Autodesk Inventor part; units mm, degrees
ref_plane "Work Plane1" through (-7, 16.75, 0) normal (0, 1, 0) x (1, 0, 0)
ref_plane "Work Plane2" through (-7, 15.75, 2) normal (0, 1, 0) x (1, 0, 0)
ref_plane "YZ Plane" through (0, 0, 0) normal (1, 0, 0) x (0, 1, 0)
sketch "Sketch1" plane through (0, 0, 0) normal (0, 0, 1) x (1, 0, 0)
  line L0 (-9.8, 0) -> (9.8, 0) construction
  line L1 (0, -20.65) -> (0, 20.65) construction
  line L2 (7, -14.75) -> (-7, -14.75)
  line L3 (-7, -14.75) -> (-7, 14.75)
  line L4 (-7, 14.75) -> (7, 14.75)
  line L5 (7, 14.75) -> (7, -14.75)
  line L6 (7, -14.75) -> (-7, 14.75) construction
  line L7 (-7, -14.75) -> (7, 14.75) construction
  point P0 (0, 0)
  dimension "d0" = 14
  dimension "d1" = 29.5
extrude "Extrusion1" add sketch "Sketch1" along normal blind 2
ref_plane "Work Plane1" through (-7, 16.75, 0) normal (0, 1, 0) x (1, 0, 0)
sketch "Sketch2" plane through (-7, 16.75, 0) normal (0, 1, 0) x (1, 0, 0)
  line L0 (0, 0) -> (14, 0) construction
  line L1 (0, 0) -> (0, -2) construction
  line L2 (14, -2) -> (0, -2) construction
  line L3 (14, 0) -> (14, -2) construction
  circle A0 centre (14, -1.5) radius 1.5
  point P0 (7, 0)
  dimension "d5" = 3
extrude "Extrusion2" add sketch "Sketch2" against normal blind 33.5
ref_plane "Work Plane2" through (-7, 15.75, 2) normal (0, 1, 0) x (1, 0, 0)
sketch "Sketch3" plane through (-7, 15.75, 2) normal (0, 1, 0) x (1, 0, 0)
  arc A0 (14, 2) -> (12.5858, 0) centre (14, 0.5) ccw construction
  line L0 (0, 2) -> (14, 2) construction
  line L1 (0, 2) -> (0, 0) construction
  line L2 (12.5858, 0) -> (0, 0) construction
  line L3 (0, 2) -> (0, 0)
  circle A1 centre (0, 0.5) radius 1.5
  point P0 (7, 2)
  dimension "d9" = 3
extrude "Extrusion3" add sketch "Sketch3" against normal blind 31.5
sketch "Skizze5" plane through (-7, 14.75, 0) normal (0, 1, 0) x (1, 0, 0)
  arc A0 (1.4142, -2) -> (0, 0) centre (0, -1.5) ccw
  line L0 (12.5858, -2) -> (1.4142, -2)
  arc A1 (14, 0) -> (12.5858, -2) centre (14, -1.5) ccw
  line L1 (0, 0) -> (14, 0)
  point P0 (7, 0)
extrude "Extrusion4" cut sketch "Skizze5" against normal blind 0.75
sketch "Skizze6" plane through (-7, -14.75, 0) normal (0, -1, 0) x (1, 0, 0)
  arc A0 (0, 0) -> (1.4142, 2) centre (0, 1.5) ccw
  line L0 (14, 0) -> (0, 0)
  arc A1 (12.5858, 2) -> (14, 0) centre (14, 1.5) ccw
  line L1 (1.4142, 2) -> (12.5858, 2)
  point P0 (7, 0)
extrude "Extrusion5" cut sketch "Skizze6" against normal blind 0.75
equation "\"d6\" = d1 + 2 * d4"
properties part number "20_Rect_Aperture_door_slide"
CAD build for the part. Positions are in the model's coordinates, mm. A direction names the side the tool comes from. Give positions to 0.01 mm unless a question says otherwise; leave off trailing zeros. Loops run counter-clockwise (first coordinate to the right, second up) from the corner with the lowest first, then second, coordinate; pieces in that order, holes last. Notation, with made-up numbers: M 50.25,29.5 L 71.25,29.5 A24 ccw 71.25,56.5 Z; hole C 25.5,42.5 d5. An arc over 180 degrees is marked long. Write each question's results on one line, items separated by ' | '.
Q1. Mould opens along X. For faces 4 (the face through (7, 16.75, 1)), 5 (the face through (0, 0, 2)), 6 (the face through (5.8, 14.4, 0.6)) say: pulls with the +X half, pulls with the -X half, needs draft (parallel to the pull), parting line crosses it, or undercut.
Geometry check:
face 4: needs draft | face 5: undercut | face 6: undercut
Q2. Which spindle directions (+Z, -Z, +X, -X, +Y, -Y) get a long thin tool onto all of the face, cutting with end or side? Do faces 1 (the face through (-5.8, -14.4, 0.6)), 2 (the face through (-7, 15.75, 1)), 3 (the face through (-7, -15.75, 1)). Say none if no direction does.
Geometry check:
face 1: -Y | face 2: +Z, -Z, -X, +Y | face 3: +Z, -Z, -X, -Y
Q3. Band-saw the part on A-A on z = 2.6. Write the cut outline in (x, y), and give its area (3 significant figures).
Geometry check:
outline: M -8.02,-15.75 L -5.98,-15.75 L -5.98,15.75 L -8.02,15.75 Z; M 5.98,-16.75 L 8.02,-16.75 L 8.02,16.75 L 5.98,16.75 Z | area: 133 mm²
Q4. Band-saw the part on D-D on y = 7.5. Write the cut outline in (x, z).
Geometry check:
outline: M -7,0 L 7,0 A1.5 ccw long 5.59,2 L -5.59,2 A1.5 ccw long Z
Q5. Flat gauge pins, fed straight in: P1, Ø6, axis at x = -0.5, y = 3.5, coming from the +Z side; P2, Ø0.9, axis at x = -6.5, z = 1.5, coming from the -Y side; P3, Ø0.6, axis at x = 1.5, z = 0.5, coming from the +Y side. Where does each tip first touch, or does it go through?
Geometry check:
P1: stops at z = 2 | P2: stops at y = -15.75 | P3: stops at y = 14
Q6. Probe probe 1 along Z at (x, y) = (-0.5, 6); probe 2 along Y at (x, z) = (0, 1.95); probe 3 along X at (y, z) = (1.5, 2.2). List the from-to ranges inside material, lowest first.
Geometry check:
probe 1: z = 0 to 2 | probe 2: y = -14 to 14 | probe 3: x = -8.33 to -5.67, 5.67 to 8.33
Q7. Band-saw the part on B-B on x = 1.5. Write the cut outline in (y, z).
Geometry check:
outline: M -14,0 L 14,0 L 14,2 L -14,2 Z
Q8. Band-saw the part on C-C on z = 0.95. Write the cut outline in (x, y).
Geometry check:
outline: M -8.4,-15.75 L -5.6,-15.75 L -5.6,-14 L 5.6,-14 L 5.6,-16.75 L 8.4,-16.75 L 8.4,16.75 L 5.6,16.75 L 5.6,14 L -5.6,14 L -5.6,15.75 L -8.4,15.75 Z
